Geometry check sheet. Reference: the model listing, model coordinates, mm. A direction names the side the tool comes from. Give positions to 0.01 mm unless a question says otherwise; leave off trailing zeros. Order: outer loops, then holes, each group sorted by start corner. A loop starts at its lowest first (then second) coordinate and runs counter-clockwise, first axis right, second up. Notation, with made-up numbers: M 43,-5.75 L 73,-5.75 A26 ccw 73,13.25 Z; hole C 19.25,37 d7. An arc over 180 degrees is marked long. Answer as CSV lines item,"result". Start each with the question number.
Q1. Thickness scan on line 1 (X direction, y = 223, z = 362.5); line 2 (X direction, y = 105, z = 399); line 3 (Z direction, x = 237, y = 215.5). Record the ranges inside material, lowest first.
Q2. Section check B-B, the plane y = 289.5. Record the boundary of the cut face in (x, z).
Q3. Section check A-A, the plane z = 463. Record the boundary of the cut face in (x, y).
Q4. Mould release check, pull along Z, two halves, no side actions. Record for faces 1 (the flat face through (-90, 395, 189)), 2 (the flat face through (-7, 197, 0)), 3 (the flat face through (426, 197, 500)): +Z half, -Z half, draft (parallel to the pull), parting line (faces both ways), or undercut.
Q5. Set-up check for faces 4 (the flat face through (-1, 395, 85)), 5 (the flat face through (-500, 197, 253)): record each of +Z, -Z, +X, -X, +Y, -Y from which the full face is reachable in a straight line by a thin tool's end or side.
Q6. Go/stop test with flat-tipped pins: pin 1 (4 mm diameter, centred on x = -169.5, y = 107.5, fed in from +Z); pin 2 (5 mm diameter, centred on x = -136.5, y = 148, fed in from +Z); pin 3 (6 mm diameter, centred on x = -94.5, z = 190.5, fed in from +Y). Record where each tip stops, or that it passes through.
Q7. Section check C-C, the plane x = 37. Record the boundary of the cut face in (y, z).
Q8. Section check D-D, the plane z = 398. Record the boundary of the cut face in (x, y).
```python
from build123d import *

# Parameters (mm, degrees)
EXTRUDE_1_DEPTH     = 400
SKETCH_2_W          = 128
SKETCH_2_H          = 72
CUT_EXTRUDE_1_DEPTH = 5
SKETCH_3_W          = 50
SKETCH_3_H          = 50
CUT_EXTRUDE_3_DEPTH = 5
SKETCH_4_W          = 20
SKETCH_4_H          = 100
CUT_EXTRUDE_4_DEPTH = 5


with BuildPart() as part:
    # 草图1 → 凸台-拉伸1 (new body)
    with BuildSketch(Plane(origin=(0, 0, 0), x_dir=(1, 0, 0), z_dir=(0, 1, 0))):
        with BuildLine():
            Line((0, 0), (500, 0))
            Line((500, 0), (500, -500))
            Line((500, -500), (350, -500))
            ThreePointArc((350, -500), (0, -266.137476728), (-350, -500))
            Line((-350, -500), (-500, -500))
            Line((-500, -500), (-500, 0))
            Line((-500, 0), (0, 0))
        make_face()
    extrude(amount=EXTRUDE_1_DEPTH)

    # 草图2 → 切除-拉伸1 (cut)
    with BuildSketch(Plane(origin=(0, 400, 0), x_dir=(1, 0, 0), z_dir=(0, 1, 0))):
        with Locations((0, -86)):
            Rectangle(SKETCH_2_W, SKETCH_2_H)
    extrude(amount=-CUT_EXTRUDE_1_DEPTH, mode=Mode.SUBTRACT)

    # 草图3 → 切除-拉伸3 (cut)
    with BuildSketch(Plane(origin=(0, 400, 0), x_dir=(1, 0, 0), z_dir=(0, 1, 0))):
        with Locations((0, -195)):
            Rectangle(SKETCH_3_W, SKETCH_3_H)
    extrude(amount=-CUT_EXTRUDE_3_DEPTH, mode=Mode.SUBTRACT)

    # 草图4 → 切除-拉伸4 (cut)
    with BuildSketch(Plane(origin=(0, 400, 0), x_dir=(1, 0, 0), z_dir=(0, 1, 0))):
        with Locations((-90, -190)):
            Rectangle(SKETCH_4_W, SKETCH_4_H)
    extrude(amount=-CUT_EXTRUDE_4_DEPTH, mode=Mode.SUBTRACT)


solid = part.part
```
Answer block:
1,line 1,"x = -500 to -252.44, 252.44 to 500"
1,line 2,"x = -500 to -288.12, 288.12 to 500"
1,line 3,"z = 0 to 349.43"
2,outline,"M -500,0 L 500,0 L 500,500 L 350,500 A378.84 cw -350,500 L -500,500 Z"
3,outline,"M -500,0 L -332.27,0 L -332.27,400 L -500,400 Z; M 332.27,0 L 500,0 L 500,400 L 332.27,400 Z"
4,face 1,"undercut"
4,face 2,"-Z half"
4,face 3,"+Z half"
5,face 4,"+Y"
5,face 5,"+Z, -Z, -X, +Y, -Y"
6,pin 1,"stops at z = 307.18"
6,pin 2,"stops at z = 292.56"
6,pin 3,"stops at y = 395"
7,outline,"M 0,0 L 400,0 L 400,50 L 395,50 L 395,122 L 400,122 L 400,267.95 L 0,267.95 Z"
8,outline,"M -500,0 L -287.26,0 L -287.26,400 L -500,400 Z; M 287.26,0 L 500,0 L 500,400 L 287.26,400 Z"
